```python
from build123d import *

# Parameters (mm, degrees)
BOSS_EXTRUDE1_DEPTH = 4
FILLET1_R           = 4.2
SKETCH3_R           = 3
SKETCH3_R_2         = 2.025
CUT_EXTRUDE1_DEPTH  = 49.76638045
SKETCH2_R           = 10
SKETCH2_R_2         = 7
BOSS_EXTRUDE2_DEPTH = 1


with BuildPart() as part:
    # Sketch1 → Boss-Extrude1 (new body)
    with BuildSketch(Plane(origin=(0, 0, 0), x_dir=(1, 0, 0), z_dir=(0, 1, 0))):
        with BuildLine():
            Line((0, -7.47801578), (0, 7.47801578))
            Line((0, 7.47801578), (21.555297549, 20.045096945))
            ThreePointArc((21.555297549, 20.045096945), (26.746562982, 19.577458446), (28.897035116, 24.325446668))
            Line((28.897035116, 24.325446668), (39.960063413, 30.775368049))
            Line((39.960063413, 30.775368049), (39.960063413, -30.775340317))
            Line((39.960063413, -30.775340317), (28.897031775, -24.325424666))
            ThreePointArc((28.897031775, -24.325424666), (26.746553125, -19.577458381), (21.555304058, -20.04508578))
            Line((21.555304058, -20.04508578), (0, -7.47801578))
        make_face()
    extrude(amount=BOSS_EXTRUDE1_DEPTH)

    # Fillet1
    fillet1_edges = [part.edges().sort_by_distance(p)[0] for p in [
        (0, 2, 7.47801578),
        (0, 2, -7.47801578),
        (21.555297549, 2, -20.045096945),
        (28.897035116, 2, -24.325446668),
        (39.960063413, 2, -30.775368049),
        (39.960063413, 2, 30.775340317),
        (28.897031775, 2, 24.325424666),
        (21.555304058, 2, 20.04508578),
    ]]
    fillet(fillet1_edges, radius=FILLET1_R)

    # Sketch3 → Cut-Extrude1 (cut, through all)
    with BuildSketch(Plane(origin=(0, 4, 0), x_dir=(1, 0, 0), z_dir=(0, 1, 0))):
        with Locations(Location((24.18, 0, 0), (0, 0, 270))):
            Circle(SKETCH3_R)
        with Locations(Location((36.06, -22.995, 0), (0, 0, 270))):
            Circle(SKETCH3_R_2)
        with Locations(Location((36.06, 22.995, 0), (0, 0, 270))):
            Circle(SKETCH3_R_2)
        with Locations(Location((4.5, 5.065, 0), (0, 0, 270))):
            Circle(SKETCH3_R_2)
        with Locations(Location((4.5, -5.065, 0), (0, 0, 270))):
            Circle(SKETCH3_R_2)
    extrude(amount=-CUT_EXTRUDE1_DEPTH, mode=Mode.SUBTRACT)

    # Sketch2 → Boss-Extrude2 (add)
    with BuildSketch(Plane(origin=(0, 4, 0), x_dir=(1, 0, 0), z_dir=(0, 1, 0))):
        with Locations(Location((24.18, 0, 0), (0, 0, 270))):
            Circle(SKETCH2_R)
        with Locations(Location((24.18, 0, 0), (0, 0, 270))):
            Circle(SKETCH2_R_2, mode=Mode.SUBTRACT)
    extrude(amount=BOSS_EXTRUDE2_DEPTH)


solid = part.part
```
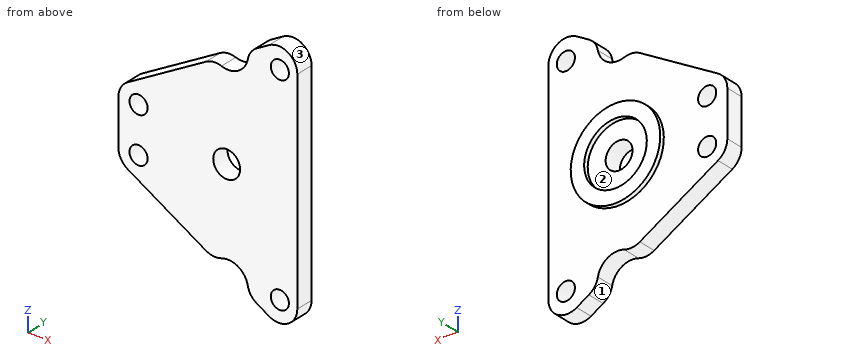
Could you check a few things on this model? Use its own coordinates, in mm. Face numbers are marked on the shaded views. Coordinates: 2 decimals unless noted, no trailing zeros. Loops run counter-clockwise (first coordinate to the right, second up) from the corner with the lowest first, then second, coordinate; pieces in that order, holes last.
1) Thinking about a two-plate mould opening in Z: for the marked faces 1, 2 and 3, which applies, released by +Z, released by -Z, zero draft, split by the parting line, or undercut?
Reported:
face 1: released by -Z
face 2: undercut
face 3: released by +Z
2) Imagine slicing it at C-C (x = 24.18). List the corners of the cut face in (y, z) for me.
Reported:
outline: (0, -18.98) - (4, -18.98) - (4, -10) - (5, -10) - (5, -7) - (4, -7) - (4, -3) - (0, -3) - close; (0, 3) - (4, 3) - (4, 7) - (5, 7) - (5, 10) - (4, 10) - (4, 18.98) - (0, 18.98) - close
3) Imagine slicing it at A-A (z = 0). List the corners of the cut face in (x, y) for me, and give its area (3 significant figures).
Reported:
outline: (0, 0) - (21.18, 0) - (21.18, 4) - (17.18, 4) - (17.18, 5) - (14.18, 5) - (14.18, 4) - (0, 4) - close; (27.18, 0) - (39.96, 0) - (39.96, 4) - (34.18, 4) - (34.18, 5) - (31.18, 5) - (31.18, 4) - (27.18, 4) - close
area: 142 mm2
4) Will these pins go through, and if not, where does the flat tip stop? pin 1 Ø4.5 at (x, z) = (36.06, -22.995) entering from +Y; pin 2 Ø4.5 at (x, z) = (4.5, -5.065) entering from -Y.
Reported:
pin 1: stops at y = 4
pin 2: stops at y = 0
5) Please list where these lines run through material, in increasing order: line 1 along Z through (x, y) = (36, 2.4); line 2 along X through (y, z) = (4.7, 0); line 3 along X through (y, z) = (2.4, 0).
Reported:
line 1: z = -27.66 to -25.02, -20.97 to 20.97, 25.02 to 27.66
line 2: x = 14.18 to 17.18, 31.18 to 34.18
line 3: x = 0 to 21.18, 27.18 to 39.96
6) Imagine slicing it at B-B (x = 36.06). List the corners of the cut face in (y, z) for me.
Reported:
outline: (0, -27.65) - (4, -27.65) - (4, -25.02) - (0, -25.02) - close; (0, -20.97) - (4, -20.97) - (4, 20.97) - (0, 20.97) - close; (0, 25.02) - (4, 25.02) - (4, 27.65) - (0, 27.65) - close
7) Imagine slicing it at D-D (y = 2.2). State how many separate pieces and enclosed holes the cut face has, and give its area (3 significant figures).
Reported:
separate pieces: 1
enclosed holes: 5
area: 1,380 mm2
